Source: CAD feature listing. Evaluate the final solid. Frame: model axes, mm. Give positions to 0.01 mm unless a question says otherwise; leave off trailing zeros. Loops run counter-clockwise (first coordinate to the right, second up) from the corner with the lowest first, then second, coordinate; pieces in that order, holes last. Notation, with made-up numbers: (43.5, 60.5) - (61.5, 60.5) arc R12 cw to (61.5, 72.5) - close; hole circle Ø11 at (-23.75, 41.5). An arc over 180 degrees is marked (long way). Put each result on its own line as item: value.
```python
from build123d import *

# Parameters (mm, degrees)
F1_DEPTH = 5
F2_R     = 5
F3_DEPTH = 389
F4_R     = 5
F5_DEPTH = 5.001


# Not quite as in the source:
# - an extrude ends at something that could not be found from the text; its depth is read off the source's solid


with BuildPart() as f1:
    # F0 (on Top) → F1 (new body)
    with BuildSketch(Plane.XY):
        with BuildLine():
            ThreePointArc((182.6944426466, 42.1886855807), (131.7434290728, 40.4795108007), (84.8448510232, 60.4657670673))
            ThreePointArc((84.8448510232, 60.4657670673), (-20.2682643936, 62.6366103984), (0, -40.5267409035))
            ThreePointArc((0, -40.5267409035), (0.8188047448, 46.5454009095), (84.8448510232, 23.7013236039))
            ThreePointArc((84.8448510232, 23.7013236039), (133.7696468349, 11.680757797), (182.6944426466, 23.7013236039))
            ThreePointArc((182.6944426466, 23.7013236039), (205.0971207079, 39.8391466865), (232.6069186924, 42.1886855807))
            ThreePointArc((232.6069186924, 42.1886855807), (207.6506806695, 65.7101106777), (182.6944426466, 42.1886855807))
        make_face()
    extrude(amount=F1_DEPTH)

    # F2 (on Top) → F3 (cut, through all)
    with BuildSketch(Plane.XY):
        with Locations((210.5412267722, 54.1418395773)):
            Circle(F2_R)
    extrude(amount=-F3_DEPTH, mode=Mode.SUBTRACT)

    # F4 (on face) → F5 (cut, through all)
    with BuildSketch(Plane.XY.offset(5)):
        with Locations((207.6506806695, 52.6958927512)):
            Circle(F4_R)
    extrude(amount=-F5_DEPTH, mode=Mode.SUBTRACT)


solid = f1.part
```
1) Material intervals for line 1 along X through (y, z) = (50, 0.45); line 2 along X through (y, z) = (49.5, 1.8); line 3 along X through (y, z) = (28.5, 0.55), sorted ascending. Write a range as [from, to].
Check result:
line 1: [-28.66, 5.96], [62.07, 102.56], [184.44, 203.44], [211.86, 230.86]
line 2: [-28.91, 5.13], [62.9, 103.62], [184.25, 203.81], [211.5, 231.05]
line 3: [-35.44, -14.55], [82.58, 187.07]
2) Section query A-A, the plane x = -7.5. Output: boundary loops of the cut face in (y, z), plus the area to 3 significant figures.
Check result:
outline: (-35.94, 0) - (-33.38, 0) - (-33.38, 5) - (-35.94, 5) - close; (38.77, 0) - (74.37, 0) - (74.37, 5) - (38.77, 5) - close
area: 191 mm²
3) Section query D-D, the plane x = 44.5. Output: boundary loops of the cut face in (y, z), plus the area to 3 significant figures.
Check result:
outline: (56.68, 0) - (85.44, 0) - (85.44, 5) - (56.68, 5) - close
area: 144 mm²
4) Pin query (flat end, axial travel): P1, Ø1.5, axis at x = 111.5, z = 3, coming from the -Y side; P2, Ø1.5, axis at y = -5.5, z = 2.5, coming from the +X side; P3, Ø9, axis at x = 207.65, y = 52.7, coming from the -Z side. Return the tip coordinate at first contact, or that it passes through.
Check result:
P1: y = 13.9
P2: x = -20.25
P3: through
5) Section query C-C, the plane z = 2.35. Output: boundary loops of the cut face in (x, y).
Check result:
outline: (0, -40.53) arc R55 cw (long way) to (84.84, 23.7) arc R105.57 ccw to (182.69, 23.7) arc R51.84 cw to (232.61, 42.19) arc R25 ccw to (182.69, 42.19) arc R117.75 cw to (84.84, 60.47) arc R67.5 ccw (long way) to start; hole circle Ø10 at (207.65, 52.7)
6) Section query B-B, the plane y = 30. Output: boundary loops of the cut face in (x, z).
Check result:
outline: (-35.22, 0) - (-13.73, 0) - (-13.73, 5) - (-35.22, 5) - close; (81.76, 0) - (188.69, 0) - (188.69, 5) - (81.76, 5) - close
7) Mould query, pull axis X, two halves, no side actions, for faces 1 (the cylindrical face through (209.96, 48.26, 2.54)), 2 (the flat face through (78, 42, 0)). Classes: pulls with the +X half, pulls with the -X half, needs draft (parallel to the pull), parting line crosses it, or undercut.
Check result:
face 1: undercut
face 2: needs draft
